Part model, mm, in its own coordinate system. Give positions to 0.01 mm unless a question says otherwise; leave off trailing zeros. Use one line per item in the form item = value. Start each with the question number.
1. Pin check, flat tips, straight feed: P1, Ø2.5, axis at x = 632.4, z = 70.26, coming from the -Y side; P2, Ø4, axis at y = 5, z = 70.5, coming from the +X side; P3, Ø5.5, axis at y = 4, z = 199, coming from the -X side; P4, Ø1, axis at x = 450.5, y = 5.5, coming from the -Z side. Stop position of each tip, or through.
2. Band-saw the part on A-A, the plane x = 438.15. State how many separate pieces and enclosed holes the cut face has, plus the area to 3 significant figures.
3. Drill centre lines: line 1 (X direction, y = 8.5, z = 150.5); line 2 (Z direction, x = 575.31, y = 6.25); line 3 (X direction, y = 9, z = 56.5). Where is each one in solid material? Low to high.
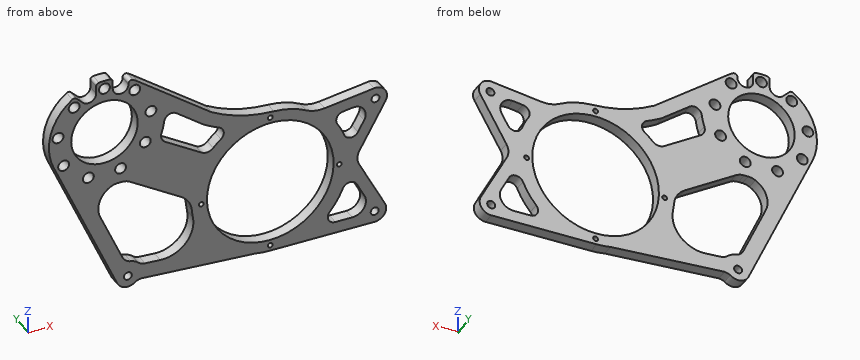
from build123d import *

# Parameters (mm, degrees)
SKETCH1_R                      = 27.4955
SKETCH1_R_2                    = 2
SKETCH1_R_3                    = 52.3875
SKETCH1_R_4                    = 3.3
BOSS_EXTRUDE1_DEPTH            = 9.525
M8_CLEARANCE_HOLE1_D           = 9
M8_CLEARANCE_HOLE1_CSINK_D     = 9.05
M8_CLEARANCE_HOLE1_CSINK_ANGLE = 90
CIRPATTERN1_COUNT              = 9
CUT_EXTRUDE2_DEPTH             = 703.782820758


with BuildPart() as part:
    # Sketch1 → Boss-Extrude1 (new body)
    with BuildSketch(Plane(origin=(0, 0, 0), x_dir=(-1, 0, 0), z_dir=(0, 1, 0))):
        with BuildLine():
            Line((-661.518109544, 9.526211138), (-574.322712035, 10.916849768))
            ThreePointArc((-574.322712035, 10.916849768), (-568.60639118, 11.272965732), (-562.947438024, 12.155797473))
            Line((-562.947438024, 12.155797473), (-468.549735034, 19.531113755))
            ThreePointArc((-468.549735034, 19.531113755), (-466.095677504, 19.039729903), (-463.807399751, 18.026003423))
            ThreePointArc((-463.807399751, 18.026003423), (-455.436670398, 15.825036693), (-448.740207572, 21.308717033))
            Line((-448.740207572, 21.308717033), (-396.041564291, 141.567674451))
            ThreePointArc((-396.041564291, 141.567674451), (-393.869824608, 172.384252636), (-411.692336104, 197.617881552))
            ThreePointArc((-411.692336104, 197.617881552), (-413.372500119, 198.071242365), (-414.950136715, 197.336701751))
            Line((-414.950136715, 197.336701751), (-420.215020333, 192.071818133))
            ThreePointArc((-420.215020333, 192.071818133), (-427.298656721, 190.662795249), (-431.31121441, 196.668012211))
            Line((-431.31121441, 196.668012211), (-431.31121441, 203.240745001))
            ThreePointArc((-431.31121441, 203.240745001), (-431.968379704, 204.945600851), (-433.59982344, 205.768273949))
            ThreePointArc((-433.59982344, 205.768273949), (-438.15, 205.994), (-442.70017656, 205.768273949))
            ThreePointArc((-442.70017656, 205.768273949), (-444.331620296, 204.945600851), (-444.98878559, 203.240745001))
            Line((-444.98878559, 203.240745001), (-444.98878559, 196.668012211))
            ThreePointArc((-444.98878559, 196.668012211), (-451.48878559, 190.168012211), (-457.98878559, 196.668012211))
            Line((-457.98878559, 196.668012211), (-457.98878559, 197.245022653))
            ThreePointArc((-457.98878559, 197.245022653), (-459.278285753, 199.455870942), (-461.837486501, 199.421924563))
            ThreePointArc((-461.837486501, 199.421924563), (-464.019895008, 198.024699819), (-466.120112298, 196.506730383))
            Line((-466.120112298, 196.506730383), (-526.629683433, 150.121113421))
            ThreePointArc((-526.629683433, 150.121113421), (-551.530592574, 139.247052869), (-578.312485484, 134.661130809))
            ThreePointArc((-578.312485484, 134.661130809), (-592.081443241, 132.419097692), (-604.99890828, 127.151270133))
            ThreePointArc((-604.99890828, 127.151270133), (-612.407574664, 124.492595217), (-620.274454537, 124.229743629))
            Line((-620.274454537, 124.229743629), (-661.161974504, 129.250099814))
            ThreePointArc((-661.161974504, 129.250099814), (-670.249252048, 125.077827159), (-670.600960367, 115.084690838))
            Line((-670.600960367, 115.084690838), (-649.049500747, 77.217685424))
            ThreePointArc((-649.049500747, 77.217685424), (-647.390214978, 71.218221534), (-648.781103624, 65.150913646))
            Line((-648.781103624, 65.150913646), (-670.149478209, 23.388671951))
            ThreePointArc((-670.149478209, 23.388671951), (-669.755736478, 14.01547017), (-661.518109544, 9.526211138))
        make_face()
        with Locations(Location((-438.15, 160.02, 0), (0, 0, 270))):
            Circle(SKETCH1_R, mode=Mode.SUBTRACT)
        with Locations(Location((-632.402453753, 70.257452317, 0), (0, 0, 270))):
            Circle(SKETCH1_R_2, mode=Mode.SUBTRACT)
        with Locations(Location((-575.31, 72.821477372, 0), (0, 0, 270))):
            Circle(SKETCH1_R_3, mode=Mode.SUBTRACT)
        with Locations(Location((-662.32278, 119.79609772, 0), (0, 0, 270))):
            Circle(SKETCH1_R_4, mode=Mode.SUBTRACT)
        with Locations(Location((-661.67, 19.05, 0), (0, 0, 270))):
            Circle(SKETCH1_R_4, mode=Mode.SUBTRACT)
        with Locations(Location((-457.464330992, 25.131712658, 0), (0, 0, 270))):
            Circle(SKETCH1_R_4, mode=Mode.SUBTRACT)
        with BuildLine():
            ThreePointArc((-518.217546247, 72.257452317), (-520.217546247, 70.257452317), (-518.217546247, 68.257452317))
            ThreePointArc((-518.217546247, 68.257452317), (-516.217546247, 70.257452317), (-518.217546247, 72.257452317))
        make_face(mode=Mode.SUBTRACT)
        with BuildLine():
            ThreePointArc((-575.31, 17.671477372), (-577.31, 15.671477372), (-575.31, 13.671477372))
            ThreePointArc((-575.31, 13.671477372), (-573.31, 15.671477372), (-575.31, 17.671477372))
        make_face(mode=Mode.SUBTRACT)
        with BuildLine():
            ThreePointArc((-575.31, 131.971477372), (-577.31, 129.971477372), (-575.31, 127.971477372))
            ThreePointArc((-575.31, 127.971477372), (-573.31, 129.971477372), (-575.31, 131.971477372))
        make_face(mode=Mode.SUBTRACT)
    extrude(amount=BOSS_EXTRUDE1_DEPTH)

    # M8 Clearance Hole1 (through all)
    with Locations(Plane(origin=(0, 0, 0), x_dir=(-1, 0, 0), z_dir=(0, -1, 0))):
        with Locations((-438.15, -199.019999978)):
            m8_clearance_hole1 = CounterSinkHole(M8_CLEARANCE_HOLE1_D / 2, M8_CLEARANCE_HOLE1_CSINK_D / 2, counter_sink_angle=M8_CLEARANCE_HOLE1_CSINK_ANGLE)

    # CirPattern1: M8 Clearance Hole1 ×9 about axis
    cirpattern1_axis = Axis((438.15, 0, 160.02), (0, 1, 0))
    for i in range(1, CIRPATTERN1_COUNT):
        add(m8_clearance_hole1.rotate(cirpattern1_axis, i * 360 / CIRPATTERN1_COUNT), mode=Mode.SUBTRACT)

    # Sketch10 → Cut-Extrude2 (cut, through all)
    with BuildSketch(Plane.XZ):
        with BuildLine():
            Line((459.226572507, 108.99771107), (501.653528527, 82.025066826))
            ThreePointArc((501.653528527, 82.025066826), (507.74174649, 75.794215969), (510.419523322, 67.504498748))
            ThreePointArc((510.419523322, 67.504498748), (510.771276342, 64.230937589), (511.288065486, 60.979343851))
            ThreePointArc((511.288065486, 60.979343851), (505.189412889, 39.365549463), (484.33326163, 31.036646412))
            Line((484.33326163, 31.036646412), (471.738439028, 32.02068307))
            ThreePointArc((471.738439028, 32.02068307), (468.684485829, 32.780789222), (466.044923926, 34.494587478))
            ThreePointArc((466.044923926, 34.494587478), (463.199383075, 36.463048748), (459.928151148, 37.590428091))
            ThreePointArc((459.928151148, 37.590428091), (455.812610468, 39.507256825), (453.051892844, 43.11146904))
            Line((453.051892844, 43.11146904), (434.678898983, 85.038868854))
            ThreePointArc((434.678898983, 85.038868854), (434.121445197, 98.905571071), (443.119806681, 109.470876354))
            ThreePointArc((443.119806681, 109.470876354), (446.028863873, 110.597089782), (449.124699442, 110.980198854))
            Line((449.124699442, 110.980198854), (452.412988142, 110.980198854))
            ThreePointArc((452.412988142, 110.980198854), (455.961057678, 110.474509108), (459.226572507, 108.99771107))
        make_face()
        with BuildLine():
            Line((488.447021855, 135.568616467), (518.5458141, 116.433517192))
            ThreePointArc((518.5458141, 116.433517192), (523.526027217, 115.31070897), (528.083819046, 117.610655627))
            ThreePointArc((528.083819046, 117.610655627), (531.194244853, 120.677331811), (534.503353276, 123.528481221))
            ThreePointArc((534.503353276, 123.528481221), (536.820485804, 129.284400418), (533.124064721, 134.267991506))
            ThreePointArc((533.124064721, 134.267991506), (526.661398117, 137.399578344), (520.391516426, 140.901217866))
            Line((520.391516426, 140.901217866), (497.676544793, 158.314132116))
            ThreePointArc((497.676544793, 158.314132116), (491.351665893, 159.127989595), (487.50938857, 154.038455032))
            ThreePointArc((487.50938857, 154.038455032), (486.663269024, 149.130057447), (485.330309415, 144.330942547))
            ThreePointArc((485.330309415, 144.330942547), (485.381225421, 139.4135911), (488.447021855, 135.568616467))
        make_face()
        with BuildLine():
            Line((635.420385908, 116.492899074), (643.506881083, 117.485795833))
            ThreePointArc((643.506881083, 117.485795833), (652.594158627, 113.313523178), (652.945866946, 103.320386857))
            Line((652.945866946, 103.320386857), (647.859361663, 94.383139612))
            ThreePointArc((647.859361663, 94.383139612), (641.819407992, 91.195500663), (636.38230144, 95.328290853))
            ThreePointArc((636.38230144, 95.328290853), (633.867295103, 101.236717058), (630.78232235, 106.868564021))
            ThreePointArc((630.78232235, 106.868564021), (630.473854175, 112.946950119), (635.420385908, 116.492899074))
        make_face()
        with BuildLine():
            Line((643.174006589, 19.344983952), (629.092422202, 19.569564558))
            ThreePointArc((629.092422202, 19.569564558), (623.393763709, 23.333521757), (624.404021839, 30.087887821))
            ThreePointArc((624.404021839, 30.087887821), (630.562532601, 38.41885687), (635.321174208, 47.621445103))
            ThreePointArc((635.321174208, 47.621445103), (640.936661153, 51.508396194), (646.828908384, 48.055353336))
            Line((646.828908384, 48.055353336), (653.243936699, 35.517854901))
            ThreePointArc((653.243936699, 35.517854901), (652.784571346, 24.582452823), (643.174006589, 19.344983952))
        make_face()
    extrude(amount=-CUT_EXTRUDE2_DEPTH, mode=Mode.SUBTRACT)


solid = part.part
From the geometry:
q1.P1 = through
q1.P2 = 647.62
q1.P3 = 409.85
q1.P4 = 18.14
q2.separate_pieces = 4
q2.enclosed_holes = 0
q2.area = 648 mm²
q3.line_1 = 393.17 to 412.36, 463.94 to 486.95, 507.87 to 526.14
q3.line_2 = 10.9 to 13.67, 17.67 to 20.43, 125.21 to 127.97, 131.97 to 134.85
q3.line_3 = 433.32 to 447.18, 511.71 to 525.53, 625.09 to 653.21
